Design review of the part built by this model. Coordinates are the model's own, in mm. A direction names the side the tool comes from. Coordinates: 2 decimals unless noted, no trailing zeros. Loops run counter-clockwise (first coordinate to the right, second up) from the corner with the lowest first, then second, coordinate; pieces in that order, holes last. Notation, with made-up numbers: (-18.75, -2.5) - (-0.75, -2.5) arc R13 cw to (-0.75, 18.5) - close; hole circle Ø2 at (26.25, 39.25). An arc over 180 degrees is marked (long way). One line per question, with ' | ' between items.
from build123d import *

# Parameters (mm, degrees)
SKETCH1_W           = 92
SKETCH1_H           = 80
BOSS_EXTRUDE1_DEPTH = 3
CUT_EXTRUDE1_DEPTH  = 62.032778079
SKETCH3_R           = 3.5
BOSS_EXTRUDE2_DEPTH = 2.8
SKETCH4_R           = 1.8
CUT_EXTRUDE2_DEPTH  = 62.234304111
SKETCH5_R           = 2.3
CUT_EXTRUDE3_DEPTH  = 62.032778079


with BuildPart() as part:
    # Sketch1 → Boss-Extrude1 (new body)
    with BuildSketch(Plane.XY):
        Rectangle(SKETCH1_W, SKETCH1_H)
    extrude(amount=BOSS_EXTRUDE1_DEPTH)

    # Sketch2 → Cut-Extrude1 (cut, through all)
    with BuildSketch(Plane.XY.offset(3)):
        Polygon((-36, 40), (0, 4), (36, 40), align=None)
        Polygon((-36, 25.857864376), (-36, -25.857864376), (-10.142135624, 0), align=None)
        Polygon((-36, -40), (0, -4), (36, -40), align=None)
        Polygon((36, 25.857864376), (36, -25.857864376), (10.142135624, 0), align=None)
    extrude(amount=-CUT_EXTRUDE1_DEPTH, mode=Mode.SUBTRACT)

    # Sketch3 → Boss-Extrude2 (add)
    with BuildSketch(Plane.XY.offset(3)):
        with Locations(Location((-41.5, 32, 0), (0, 0, 180))):
            Circle(SKETCH3_R)
        with Locations(Location((-41.5, -16.4, 0), (0, 0, 180))):
            Circle(SKETCH3_R)
        with Locations(Location((41.5, -16.4, 0), (0, 0, 180))):
            Circle(SKETCH3_R)
        with Locations(Location((41.5, 32, 0), (0, 0, 180))):
            Circle(SKETCH3_R)
    extrude(amount=BOSS_EXTRUDE2_DEPTH)

    # Sketch4 → Cut-Extrude2 (cut, through all)
    with BuildSketch(Plane.XY.offset(5.8)):
        with Locations((-41.5, 32)):
            Circle(SKETCH4_R)
        with Locations((41.5, 32)):
            Circle(SKETCH4_R)
        with Locations((41.5, -16.4)):
            Circle(SKETCH4_R)
    extrude(amount=-CUT_EXTRUDE2_DEPTH, mode=Mode.SUBTRACT)

    # Sketch5 → Cut-Extrude3 (cut, through all)
    with BuildSketch(Plane.XY.offset(3)):
        with Locations((-40, -30)):
            Circle(SKETCH5_R)
        with Locations((40, -30)):
            Circle(SKETCH5_R)
    extrude(amount=-CUT_EXTRUDE3_DEPTH, mode=Mode.SUBTRACT)


solid = part.part
Q1. Tool access review of faces 1 (the flat face through (36, 0, 2)), 2 (the cylindrical face through (44.08, 29.635, 4.38)), 3 (the flat face through (18, -22, 2)): name each direction out of +Z, -Z, +X, -X, +Y, -Y from which nothing blocks a thin tool from reaching the whole face with its end or side.
Returned:
face 1: +Z, -Z | face 2: +Z | face 3: +Z, -Z, -Y
Q2. To check wall thickness, follow line 1 along Y through (x, z) = (41.5, 2.65); line 2 along X through (y, z) = (-9, 0.3); line 3 along X through (y, z) = (21, 2.55). State the ranges of each line that lie inside material, in increasing order.
Returned:
line 1: y = -40 to -31.74, -28.26 to -18.2, -14.6 to 30.2, 33.8 to 40 | line 2: x = -46 to -36, -19.14 to -5, 5 to 19.14, 36 to 46 | line 3: x = -46 to -36, -31.14 to -17, 17 to 31.14, 36 to 46
Q3. Take a section at D-D (x = -12.5). Give the boundary of the cut face in (y, z).
Returned:
outline: (-16.5, 0) - (-2.36, 0) - (-2.36, 3) - (-16.5, 3) - close; (2.36, 0) - (16.5, 0) - (16.5, 3) - (2.36, 3) - close
Q4. For pin 1 (7.5 mm diameter, centred on x = -40, y = -30, fed in from +Z); pin 2 (3 mm diameter, centred on x = 0.5, z = 1.5, fed in from -Y); pin 3 (1 mm diameter, centred on x = -10, z = 2, fed in from +Y), all flat-tipped, find the tip position at first contact; note any pin that passes through.
Returned:
pin 1: stops at z = 3 | pin 2: stops at y = -6 | pin 3: stops at y = 14.5
Q5. Take a section at C-C (y = -1). Give the boundary of the cut face in (x, z).
Returned:
outline: (-46, 0) - (-36, 0) - (-36, 3) - (-46, 3) - close; (-11.14, 0) - (11.14, 0) - (11.14, 3) - (-11.14, 3) - close; (36, 0) - (46, 0) - (46, 3) - (36, 3) - close
Q6. Take a section at B-B (y = 20). Give the boundary of the cut face in (x, z), plus the area to 3 significant figures.
Returned:
outline: (-46, 0) - (-36, 0) - (-36, 3) - (-46, 3) - close; (-30.14, 0) - (-16, 0) - (-16, 3) - (-30.14, 3) - close; (16, 0) - (30.14, 0) - (30.14, 3) - (16, 3) - close; (36, 0) - (46, 0) - (46, 3) - (36, 3) - close | area: 145 mm²
Q7. Draft analysis for pull direction X (two halves, no side actions). For faces 4 (the flat face through (-41, 30, 5.8)), 5 (the flat face through (-36, 0, 2)), 6 (the flat face through (-18, -22, 2)), 7 (the flat face through (-46, -1, 1)), state which applies: +X half, -X half, draft (parallel to the pull), parting line (faces both ways), or undercut.
Returned:
face 4: draft | face 5: undercut | face 6: undercut | face 7: -X half
Q8. Take a section at A-A (z = 4.1). Give the boundary of the cut face in (x, y).
Returned:
outline: circle Ø7 at (-41.5, -16.4); circle Ø7 at (-41.5, 32); circle Ø7 at (41.5, -16.4); circle Ø7 at (41.5, 32); hole circle Ø3.6 at (-41.5, 32); hole circle Ø3.6 at (41.5, -16.4); hole circle Ø3.6 at (41.5, 32)
